from build123d import *

# Parameters (mm, degrees)
SKETCH1_W          = 55
SKETCH1_H          = 28
PCB_DEPTH          = 1.6
WROOM_SHIELD_START = 1.6
SKETCH2_W          = 18
SKETCH2_H          = 25.5
WROOM_SHIELD_DEPTH = 3
MICRO_USB_START    = 1.6
SKETCH3_W          = 6
SKETCH3_H          = 8
MICRO_USB_DEPTH    = 3
HEADER_1_START     = 1.6
SKETCH4_W          = 38
SKETCH4_H          = 2.5
HEADER_1_DEPTH     = 2.5
HEADER_2_START     = 1.6
SKETCH5_W          = 38
SKETCH5_H          = 2.5
HEADER_2_DEPTH     = 2.5
BUTTON_EN_START    = 1.6
SKETCH6_W          = 4
SKETCH6_H          = 3
BUTTON_EN_DEPTH    = 1.5


with BuildPart() as part:
    # Sketch1 → PCB (new body)
    with BuildSketch(Plane(origin=(0, 0, 0), x_dir=(1, 0, 0), z_dir=(0, 1, 0))):
        Rectangle(SKETCH1_W, SKETCH1_H)
    extrude(amount=PCB_DEPTH)

    # Sketch2 → WROOM_Shield (add)
    with BuildSketch(Plane(origin=(0, 0, 0), x_dir=(1, 0, 0), z_dir=(0, 1, 0)).offset(WROOM_SHIELD_START)):
        with Locations((17.5, 0)):
            Rectangle(SKETCH2_W, SKETCH2_H)
    extrude(amount=WROOM_SHIELD_DEPTH)

    # Sketch3 → Micro_USB (add)
    with BuildSketch(Plane(origin=(0, 0, 0), x_dir=(1, 0, 0), z_dir=(0, 1, 0)).offset(MICRO_USB_START)):
        with Locations((-24.5, 0)):
            Rectangle(SKETCH3_W, SKETCH3_H)
    extrude(amount=MICRO_USB_DEPTH)

    # Sketch4 → Header_1 (add)
    with BuildSketch(Plane(origin=(0, 0, 0), x_dir=(1, 0, 0), z_dir=(0, 1, 0)).offset(HEADER_1_START)):
        with Locations((-5, -12.5)):
            Rectangle(SKETCH4_W, SKETCH4_H)
    extrude(amount=HEADER_1_DEPTH)

    # Sketch5 → Header_2 (add)
    with BuildSketch(Plane(origin=(0, 0, 0), x_dir=(1, 0, 0), z_dir=(0, 1, 0)).offset(HEADER_2_START)):
        with Locations((-5, 12.5)):
            Rectangle(SKETCH5_W, SKETCH5_H)
    extrude(amount=HEADER_2_DEPTH)

    # Sketch6 → Button_EN (add)
    with BuildSketch(Plane(origin=(0, 0, 0), x_dir=(1, 0, 0), z_dir=(0, 1, 0)).offset(BUTTON_EN_START)):
        with Locations((-15.5, -7)):
            Rectangle(SKETCH6_W, SKETCH6_H)
    extrude(amount=BUTTON_EN_DEPTH)


solid = part.part
Work out the finished part from the listing and answer in its coordinate system (mm). A direction names the side the tool comes from. Give positions to 0.01 mm unless a question says otherwise; leave off trailing zeros. Write each loop counter-clockwise with the first axis right and the second up, starting at its lowest first coordinate (ties: lowest second). Pieces come first, ordered by that corner, then holes.
Q1. The part is cut by section C-C on x = -9.5. Give the vertices of the cut face in (y, z).
Answer:
outline: (0, -14) - (1.6, -14) - (1.6, -13.75) - (4.1, -13.75) - (4.1, -11.25) - (1.6, -11.25) - (1.6, 11.25) - (4.1, 11.25) - (4.1, 13.75) - (1.6, 13.75) - (1.6, 14) - (0, 14) - close
Q2. The part is cut by section B-B on z = 6. Give the vertices of the cut face in (x, y), and give its area (3 significant figures).
Answer:
outline: (-27.5, 0) - (27.5, 0) - (27.5, 1.6) - (26.5, 1.6) - (26.5, 4.6) - (8.5, 4.6) - (8.5, 1.6) - (-13.5, 1.6) - (-13.5, 3.1) - (-17.5, 3.1) - (-17.5, 1.6) - (-27.5, 1.6) - close
area: 148 mm2
Q3. Given pin 1 (2 mm diameter, centred on y = 2, z = 11, fed in from +X); pin 2 (1 mm diameter, centred on x = -16, z = -1, fed in from +Y); pin 3 (1.5 mm diameter, centred on y = 3.5, z = -4, fed in from +X); pin 4 (0.7 mm diameter, centred on x = -2, y = 3, fed in from +Z), each flat-ended and moving along its own axis, determine where each tip first touches the part or whether it passes through.
Answer:
pin 1: stops at x = 27.5
pin 2: stops at y = 1.6
pin 3: stops at x = 26.5
pin 4: stops at z = 13.75
Q4. A tool of negligible diameter and unlimited length cuts with its end or side. For faces 5 (the face through (-5, 3, -13.75)), 6 (the face through (-8, 3, -11.25)), 7 (the face through (8.5, 3, 0)), 8 (the face through (14, 3, 13)), from which of +Z, -Z, +X, -X, +Y, -Y can it reach the whole face along a straight path? Write none if from no direction.
Answer:
face 5: -Z, +X, -X, +Y
face 6: -X, +Y
face 7: +Y
face 8: +Z, +X, +Y
Q5. The part is cut by section A-A on x = 18. Give the vertices of the cut face in (y, z).
Answer:
outline: (0, -14) - (1.6, -14) - (1.6, -12.75) - (4.6, -12.75) - (4.6, 12.75) - (1.6, 12.75) - (1.6, 14) - (0, 14) - close
Q6. The part is cut by section D-D on z = -5.75. Give the vertices of the cut face in (x, y), and give its area (3 significant figures).
Answer:
outline: (-27.5, 0) - (27.5, 0) - (27.5, 1.6) - (26.5, 1.6) - (26.5, 4.6) - (8.5, 4.6) - (8.5, 1.6) - (-27.5, 1.6) - close
area: 142 mm2
Q7. Straight lines are drawn through the part: L1, parallel to X at y = 2.1, z = -1.5; L2, parallel to X at y = 2.15, z = 6.75; L3, parallel to Z at x = -8, y = 3.85. For each, find the intervals that lie inside material, in ascending order.
Answer:
L1: x = -27.5 to -21.5, 8.5 to 26.5
L2: x = -17.5 to -13.5, 8.5 to 26.5
L3: z = -13.75 to -11.25, 11.25 to 13.75
Q8. For a pull along Z with two mould halves and no side action, classify faces 1 (the face through (0, 0, 0)), 2 (the face through (-13.5, 2, 7)), 3 (the face through (-16, 3.1, 7)), 4 (the face through (0, 1, -14)) as released by +Z, released by -Z, zero draft, split by the parting line, or undercut.
Answer:
face 1: zero draft
face 2: undercut
face 3: undercut
face 4: released by -Z
